```python
from build123d import *

# Parameters (mm, degrees)
SKETCH005_W     = 71
SKETCH005_H     = 76.2
PAD_DEPTH       = 22
SKETCH003_R     = 11.5
SKETCH003_R_2   = 3.1
POCKET_DEPTH    = 30
SKETCH004_R     = 4.15
POCKET001_DEPTH = 16
SKETCH_R        = 6
POCKET002_DEPTH = 6


with BuildPart() as part:
    # Sketch005 → Pad (new body)
    with BuildSketch(Plane.YZ):
        with Locations((-35.5, 38.1)):
            Rectangle(SKETCH005_W, SKETCH005_H)
    extrude(amount=PAD_DEPTH)

    # Sketch003 → Pocket (cut)
    with BuildSketch(Plane.YZ.offset(22)):
        with Locations((-37.5, 38.1)):
            Circle(SKETCH003_R)
        with Locations((-25, 16.449365)):
            Circle(SKETCH003_R_2)
        with Locations((-25, 59.750635)):
            Circle(SKETCH003_R_2)
        with Locations((-62.5, 38.1)):
            Circle(SKETCH003_R_2)
    extrude(amount=-POCKET_DEPTH, mode=Mode.SUBTRACT)

    # Sketch004 → Pocket001 (cut)
    with BuildSketch(Plane.ZX):
        with Locations((10, 8)):
            Circle(SKETCH004_R)
        with Locations((66.2, 8)):
            Circle(SKETCH004_R)
        with Locations((38.1, 15)):
            Circle(SKETCH004_R)
    extrude(amount=-POCKET001_DEPTH, mode=Mode.SUBTRACT)

    # Sketch → Pocket002 (cut)
    with BuildSketch(Plane(origin=(0, 0, 0), x_dir=(0, 1, 0), z_dir=(-1, 0, 0))):
        with Locations((-25, -59.750635)):
            Circle(SKETCH_R)
        with Locations((-25, -16.449365)):
            Circle(SKETCH_R)
        with Locations((-62.5, -38.1)):
            Circle(SKETCH_R)
    extrude(amount=-POCKET002_DEPTH, mode=Mode.SUBTRACT)


solid = part.part
```
Work out the finished part from the listing and answer in its coordinate system (mm). A direction names the side the tool comes from. Coordinates: 2 decimals unless noted, no trailing zeros. Write each loop counter-clockwise with the first axis right and the second up, starting at its lowest first coordinate (ties: lowest second). Pieces come first, ordered by that corner, then holes.
Q1. A cutting plane is placed at C-C, the plane z = 17.5. Give the vertices of the cut face in (x, y), then the cut area to 3 significant figures.
Q2. Determine the mould class of faces 1 (the face through (8.182, -7.888, 62.054)), 2 (the face through (22, -28, 47)), 3 (the face through (11, -36, 76.2)) for opening direction X: released by +X, released by -X, zero draft, split by the parting line, or undercut.
Q3. Which of the six approach directions +Z, -Z, +X, -X, +Y, -Y give full straight-line access (tool end or side, diameter ignored) to faces 4 (the face through (14.11, -60.83, 40.71)), 5 (the face through (8, -16, 10)), 6 (the face through (2.958, -68.494, 37.836))?
Q4. A cutting plane is placed at A-A, the plane z = 38.1. Give the vertices of the cut face in (x, y).
Q5. Find the intervals of material crossed by line 1 (Z direction, x = 1.45, y = -25); line 2 (Z direction, x = 18, y = -25); line 3 (Z direction, x = 3.85, y = -62.5), in increasing order.
Q6. A cutting plane is placed at D-D, the plane x = 18.25. Give the vertices of the cut face in (y, z).
Q7. A cutting plane is placed at B-B, the plane y = -24.5. Give the vertices of the cut face in (x, z).
Q8. Each of these flat-tipped pins is pushed along its axis until it touches: pin 1 Ø3.5 at (y, z) = (-25.5, 14) entering from -X; pin 2 Ø7.5 at (x, z) = (15, 38.1) entering from +Y. Where does it stop, or does it pass through?
Findings below:
1. outline: (0, -71) - (22, -71) - (22, -27.92) - (6, -27.92) - (6, -30.91) - (0, -30.91) - close; (0, -19.09) - (6, -19.09) - (6, -22.08) - (22, -22.08) - (22, 0) - (0, 0) - close
1. area: 1,400 mm2
2. face 1: undercut
2. face 2: released by +X
2. face 3: zero draft
3. face 4: +X, -X
3. face 5: +Y
3. face 6: -X
4. outline: (0, -71) - (22, -71) - (22, -65.6) - (6, -65.6) - (6, -68.5) - (0, -68.5) - close; (0, -56.5) - (6, -56.5) - (6, -59.4) - (22, -59.4) - (22, -49) - (0, -49) - close; (0, -26) - (22, -26) - (22, 0) - (19.15, 0) - (19.15, -16) - (10.85, -16) - (10.85, 0) - (0, 0) - close
5. line 1: z = 0 to 10.45, 22.45 to 53.75, 65.75 to 76.2
5. line 2: z = 0 to 13.35, 19.55 to 56.65, 62.85 to 76.2
5. line 3: z = 0 to 32.1, 44.1 to 76.2
6. outline: (-71, 0) - (0, 0) - (0, 35.52) - (-16, 35.52) - (-16, 40.68) - (0, 40.68) - (0, 76.2) - (-71, 76.2) - close; hole circle Ø6.2 at (-62.5, 38.1); hole circle Ø23 at (-37.5, 38.1); hole circle Ø6.2 at (-25, 16.45); hole circle Ø6.2 at (-25, 59.75)
7. outline: (0, 0) - (22, 0) - (22, 13.39) - (6, 13.39) - (6, 10.47) - (0, 10.47) - close; (0, 22.43) - (6, 22.43) - (6, 19.51) - (22, 19.51) - (22, 56.69) - (6, 56.69) - (6, 53.77) - (0, 53.77) - close; (0, 65.73) - (6, 65.73) - (6, 62.81) - (22, 62.81) - (22, 76.2) - (0, 76.2) - close
8. pin 1: stops at x = 6
8. pin 2: stops at y = -16
